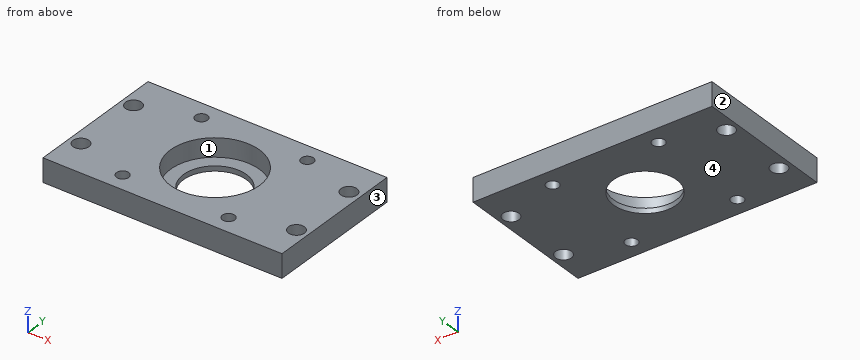
Autodesk Inventor part; units mm, degrees
ref_plane "YZ Plane" through (0, 0, 0) normal (1, 0, 0) x (0, 1, 0)
ref_plane "XZ Plane" through (0, 0, 0) normal (0, 1, 0) x (-1, 0, 0)
ref_plane "XY Plane" through (0, 0, 0) normal (0, 0, 1) x (1, 0, 0)
sketch "Sketch1" plane through (0, 0, 0) normal (0, 0, 1) x (1, 0, 0)
  line L0 (-32.2263, -19.05) -> (32.2263, -19.05)
  line L1 (32.2263, -19.05) -> (32.2263, 19.05)
  line L2 (32.2263, 19.05) -> (-32.2263, 19.05)
  line L3 (-32.2263, 19.05) -> (-32.2263, -19.05)
  line L4 (-32.2263, -19.05) -> (32.2263, 19.05) construction
  line L5 (32.2263, -19.05) -> (-32.2263, 19.05) construction
  line L6 (-25.8762, 19.05) -> (-25.8762, -19.05) construction
  line L7 (25.8762, 19.05) -> (25.8762, -19.05) construction
  line L8 (-29.0512, 19.05) -> (-29.0512, -19.05) construction
  line L9 (29.0512, 19.05) -> (29.0512, -19.05) construction
  line L10 (-32.2263, 0) -> (32.2263, 0) construction
  circle A0 centre (0, 0) radius 12
  circle A1 centre (0, 0) radius 8.5
  line L11 (-17.4625, -17.4625) -> (17.4625, -17.4625) construction
  line L12 (17.4625, -17.4625) -> (17.4625, 17.4625) construction
  line L13 (17.4625, 17.4625) -> (-17.4625, 17.4625) construction
  line L14 (-17.4625, 17.4625) -> (-17.4625, -17.4625) construction
  line L15 (-17.4625, -17.4625) -> (17.4625, 17.4625) construction
  line L16 (17.4625, -17.4625) -> (-17.4625, 17.4625) construction
  circle A2 centre (-14.2875, 14.2875) radius 3.175 construction
  line L17 (14.2875, -14.2875) -> (-14.2875, -14.2875) construction
  line L18 (-14.2875, -14.2875) -> (-14.2875, 14.2875) construction
  line L19 (-14.2875, 14.2875) -> (14.2875, 14.2875) construction
  line L20 (14.2875, 14.2875) -> (14.2875, -14.2875) construction
  line L21 (14.2875, -14.2875) -> (-14.2875, 14.2875) construction
  line L22 (-14.2875, -14.2875) -> (14.2875, 14.2875) construction
  point P0 (-29.0513, 9.525)
  point P1 (-29.0513, -9.525)
  point P2 (29.0512, -9.525)
  point P3 (29.0512, 9.525)
  dimension "d0" = 64.4525
  dimension "d1" = 38.1
  dimension "d2" = 6.35
  dimension "d3" = 6.35
  dimension "d4" = 9.525
  dimension "d5" = 9.525
  dimension "d6" = 24
  dimension "d18" = 17
  dimension "d19" = 34.925
  dimension "d20" = 34.925
  dimension "d21" = 6.35
extrude "Extrusion1" add sketch "Sketch1" against normal blind 6.35 contours L3 L2 L1 L0 | A0
hole "Hole1" at (-29.0513, 9.525, 0) at (-29.0513, -9.525, 0) at (29.0512, -9.525, 0) at (29.0512, 9.525, 0) direction (0, 0, -1) diameter 4.318 end through all
extrude "Extrusion2" cut sketch "Sketch1" against normal blind 5 contours A0 | A1
hole "Hole2" at (-14.2875, 14.2875, 0) at (-14.2875, -14.2875, 0) at (14.2875, -14.2875, 0) at (14.2875, 14.2875, 0) direction (0, 0, -1) diameter 3.302 end through all
equation "\"d20\" = d19"
properties part number "Module Top Plate" material "Aluminum 6061"
Source: CAD feature listing. Evaluate the final solid. Frame: model axes, mm. Face numbers are marked on the shaded views. Round coordinates to 2 decimals unless told otherwise and drop trailing zeros. Loops run counter-clockwise (first coordinate to the right, second up) from the corner with the lowest first, then second, coordinate; pieces in that order, holes last. Notation, with made-up numbers: (59.25, 3) - (70.25, 3) arc R16 ccw to (70.25, 33) - close; hole circle Ø3 at (20.5, 42.5). An arc over 180 degrees is marked (long way). Use CSV: the item, a comma, the result in double quotes.
Q1. Section query C-C, the plane z = -3.25. Give the number of separate pieces and of enclosed holes in the cut face, then the cut area to 3 significant figures.
Reported:
separate pieces,"1"
enclosed holes,"9"
area,"1,910 mm^2"
Q2. Section query B-B, the plane y = 0. Output: boundary loops of the cut face in (x, z).
Reported:
outline,"(-32.23, -6.35) - (-8.5, -6.35) - (-8.5, -5) - (-12, -5) - (-12, 0) - (-32.23, 0) - close; (8.5, -6.35) - (32.23, -6.35) - (32.23, 0) - (12, 0) - (12, -5) - (8.5, -5) - close"
Q3. Ray query, line 1 along X through (y, z) = (-14.5, -5.5); line 2 along X through (y, z) = (-13.5, -1.5); line 3 along X through (y, z) = (9.5, -3.25). Return the intervals inside material, ascending.
Reported:
line 1,"-32.23 to -15.92, -12.65 to 12.65, 15.92 to 32.23"
line 2,"-32.23 to -15.74, -12.84 to 12.84, 15.74 to 32.23"
line 3,"-32.23 to -31.21, -26.89 to -7.33, 7.33 to 26.89, 31.21 to 32.23"
Q4. Section query D-D, the plane y = -9.5. Output: boundary loops of the cut face in (x, z), then the cut area to 3 significant figures.
Reported:
outline,"(-32.23, -6.35) - (-31.21, -6.35) - (-31.21, 0) - (-32.23, 0) - close; (-26.89, -6.35) - (26.89, -6.35) - (26.89, 0) - (7.33, 0) - (7.33, -5) - (-7.33, -5) - (-7.33, 0) - (-26.89, 0) - close; (31.21, -6.35) - (32.23, -6.35) - (32.23, 0) - (31.21, 0) - close"
area,"281 mm^2"
Q5. Pin query (flat end, axial travel): pin 1 Ø3 at (x, y) = (-3.5, 7.5) entering from +Z; pin 2 Ø1.5 at (x, y) = (15.5, 2) entering from +Z; pin 3 Ø4 at (x, y) = (29.05, 9.52) entering from -Z. Return the tip coordinate at first contact, or that it passes through.
Reported:
pin 1,"z = -5"
pin 2,"z = 0"
pin 3,"through"
Q6. Mould query, pull axis X, two halves, no side actions, for the marked faces 1, 2, 3 and 4. Classes: pulls with the +X half, pulls with the -X half, needs draft (parallel to the pull), parting line crosses it, or undercut.
Reported:
face 1,"undercut"
face 2,"pulls with the -X half"
face 3,"pulls with the +X half"
face 4,"needs draft"
Q7. Section query A-A, the plane x = 0. Output: boundary loops of the cut face in (y, z), then the cut area to 3 significant figures.
Reported:
outline,"(-19.05, -6.35) - (-8.5, -6.35) - (-8.5, -5) - (-12, -5) - (-12, 0) - (-19.05, 0) - close; (8.5, -6.35) - (19.05, -6.35) - (19.05, 0) - (12, 0) - (12, -5) - (8.5, -5) - close"
area,"99.0 mm^2"
